Design review of the part shown in the three views and the two pictorial views. Dimensions are in mm from the part's minimum x, y and z. Coordinates: 2 decimals unless noted, no trailing zeros. Write each loop counter-clockwise with the first axis right and the second up, starting at its lowest first coordinate (ties: lowest second). Pieces come first, ordered by that corner, then holes. Notation, with made-up numbers: (-29, 49.25) -> (25, 49.25) arc R21 ccw to (25, 57.25) -> close; hole circle Ø3 at (-26, 38). An arc over 180 degrees is marked (long way). Write each question's results on one line, items separated by ' | '.
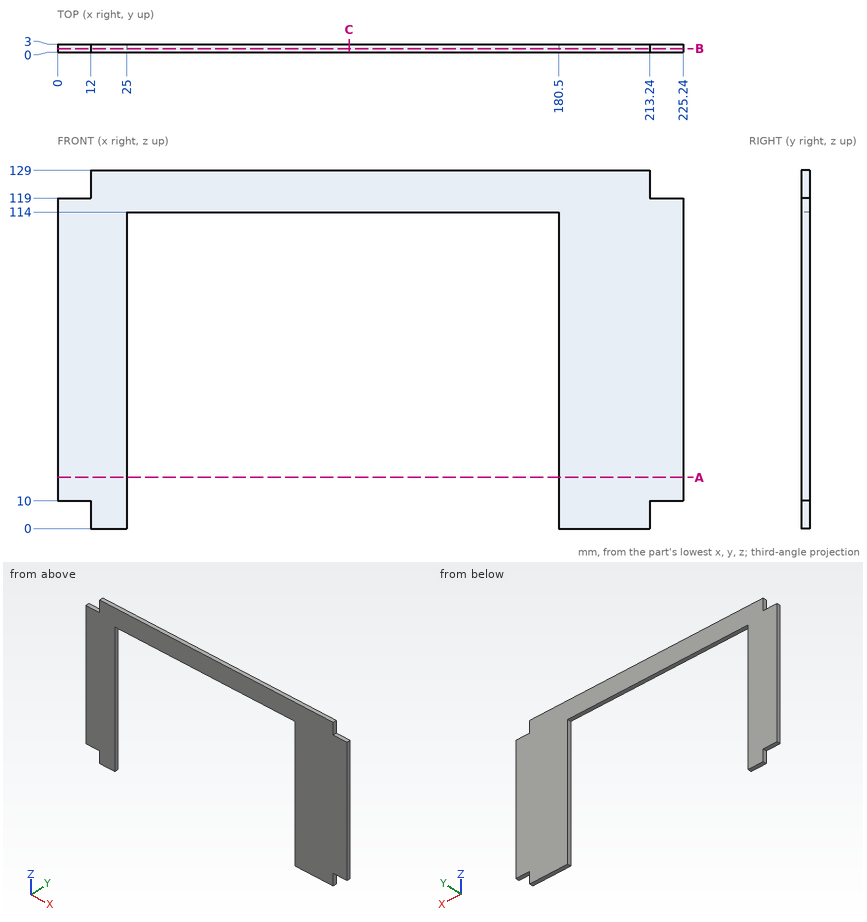
Q1. Add section A-A (z = 18.5). Write out the cut boundary in (x, y), plus the area to 3 significant figures.
Solution:
outline: (0, 0) -> (25, 0) -> (25, 3) -> (0, 3) -> close; (180.5, 0) -> (225.24, 0) -> (225.24, 3) -> (180.5, 3) -> close | area: 209 mm²
Q2. For line 1 (X direction, y = 0.1, z = 48.5); line 2 (X direction, y = 1.25, z = 6); line 3 (Z direction, x = 166, y = 1.4), list the stretches that pass through material, from the lowest coordinate up. Write a range as from..to.
Solution:
line 1: 0..25, 180.5..225.24 | line 2: 12..25, 180.5..213.24 | line 3: 114..129
Q3. Add section C-C (x = 105). Write out the cut boundary in (y, z).
Solution:
outline: (0, 114) -> (3, 114) -> (3, 129) -> (0, 129) -> close
Q4. Clearance check with flat-ended pins moving along their axes: P1, Ø0.9, axis at x = 124.5, y = 1.5, coming from the -Z side; P2, Ø0.9, axis at y = 2, z = 5, coming from the -X side; P3, Ø1.5, axis at x = 218.5, y = 1.5, coming from the +Z side. State where each tip first meets the part, or that it passes through.
Solution:
P1: z = 114 | P2: x = 12 | P3: z = 119
Q5. Add section B-B (y = 1.3). Write out the cut boundary in (x, z), plus the area to 3 significant figures.
Solution:
outline: (0, 10) -> (12, 10) -> (12, 0) -> (25, 0) -> (25, 114) -> (180.5, 114) -> (180.5, 0) -> (213.24, 0) -> (213.24, 10) -> (225.24, 10) -> (225.24, 119) -> (213.24, 119) -> (213.24, 129) -> (12, 129) -> (12, 119) -> (0, 119) -> close | area: 10,800 mm²
